Drawing for the job (mm, zero at the part's lowest x, y, z). Coordinates: 2 decimals unless noted, no trailing zeros. Write each loop counter-clockwise with the first axis right and the second up, starting at its lowest first coordinate (ties: lowest second). Pieces come first, ordered by that corner, then holes. Notation, with made-up numbers: (39.25, 73.5) - (58.25, 73.5) arc R8 ccw to (58.25, 81.5) - close; hole circle Ø2 at (1, 69.5). An arc over 180 degrees is marked (long way). Write each question's results on one line, items separated by ' | '.
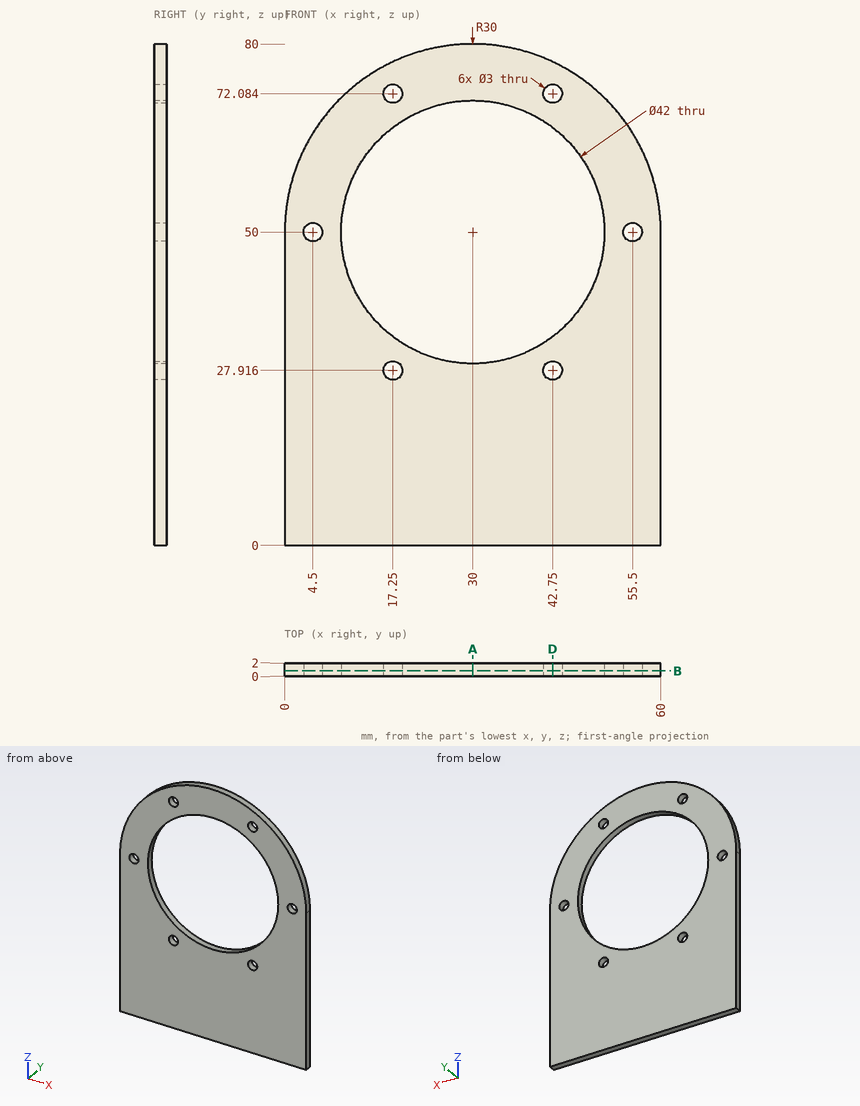
(1) Flat gauge pin, fed straight in: P1, Ø3.5, axis at x = 42.75, z = 27.92, coming from the +Y side. Where does the tip first touch, or does it go through?
Return value:
P1: stops at y = 2
(2) Saw through at B-B on y = 0.8. Write the cut outline in (x, z).
Return value:
outline: (0, 0) - (60, 0) - (60, 50) arc R30 ccw to (0, 50) - close; hole circle Ø3 at (4.5, 50); hole circle Ø42 at (30, 50); hole circle Ø3 at (17.25, 27.92); hole circle Ø3 at (17.25, 72.08); hole circle Ø3 at (42.75, 27.92); hole circle Ø3 at (42.75, 72.08); hole circle Ø3 at (55.5, 50)
(3) Saw through at D-D on x = 42.75. Write the cut outline in (y, z).
Return value:
outline: (0, 0) - (2, 0) - (2, 26.42) - (0, 26.42) - close; (0, 29.42) - (2, 29.42) - (2, 33.31) - (0, 33.31) - close; (0, 66.69) - (2, 66.69) - (2, 70.58) - (0, 70.58) - close; (0, 73.58) - (2, 73.58) - (2, 77.16) - (0, 77.16) - close
(4) Wall check: line 1 (Z direction, x = 43.5, y = 0.45) (1 decimal); line 2 (X direction, y = 0.7, z = 50); line 3 (X direction, y = 0.75, z = 28.5). Give the ranges that are in metal, low to high. Write a range as from..to.
Return value:
line 1: z = 0..26.6, 29.2..33.9, 66.1..70.8, 73.4..76.8 | line 2: x = 0..3, 6..9, 51..54, 57..60 | line 3: x = 0..15.87, 18.63..41.37, 44.13..60
(5) Saw through at A-A on x = 30. Write the cut outline in (y, z).
Return value:
outline: (0, 0) - (2, 0) - (2, 29) - (0, 29) - close; (0, 71) - (2, 71) - (2, 80) - (0, 80) - close
